Input: part model. Units: mm. Frame: model coordinates. Round coordinates to 2 decimals unless told otherwise and drop trailing zeros. Write each loop counter-clockwise with the first axis right and the second up, starting at its lowest first coordinate (ties: lowest second). Pieces come first, ordered by that corner, then holes. Notation, with made-up numbers: (-1.75, 45.5) - (44.25, 45.5) arc R13 ccw to (44.25, 59.5) - close; hole circle Ø6 at (63, 82.5). An arc over 180 degrees is marked (long way). Use one line per item in the form item = value.
```python
from build123d import *

# Parameters (mm, degrees)
BOSS_EXTRUDE1_DEPTH = 3.175
FILLET1_R           = 50.8
SKETCH2_R           = 3.175
CUT_EXTRUDE1_DEPTH  = 131.731020699
SKETCH3_R           = 2.38125
CUT_EXTRUDE2_DEPTH  = 131.731020699
SKETCH4_W           = 148.329762774
SKETCH4_H           = 42.508472293
CUT_EXTRUDE3_DEPTH  = 131.731020699


with BuildPart() as part:
    # Sketch1 → Boss-Extrude1 (new body)
    with BuildSketch(Plane.XY):
        Polygon((12.7, -76.2), (12.7, 25.4), (-25.408227408, 101.6), (-82.206807187, 101.6), (-12.7, -37.383601913), (-12.7, -76.2), align=None)
    extrude(amount=BOSS_EXTRUDE1_DEPTH)

    # Fillet1
    fillet1_edges = [part.edges().sort_by_distance(p)[0] for p in [
        (-12.7, -37.383601913, 1.5875),
    ]]
    fillet(fillet1_edges, radius=FILLET1_R)

    # Sketch2 → Cut-Extrude1 (cut, through all)
    with BuildSketch(Plane(origin=(0, 0, 0), x_dir=(-1, 0, 0), z_dir=(0, 0, -1))):
        with Locations((0, -63.5)):
            Circle(SKETCH2_R)
        with Locations((0, -38.1)):
            Circle(SKETCH2_R)
        with Locations((0, -12.7)):
            Circle(SKETCH2_R)
        with Locations((0, 12.7)):
            Circle(SKETCH2_R)
    extrude(amount=-CUT_EXTRUDE1_DEPTH, mode=Mode.SUBTRACT)

    # Sketch3 → Cut-Extrude2 (cut, through all)
    with BuildSketch(Plane(origin=(0, 0, 0), x_dir=(-1, 0, 0), z_dir=(0, 0, -1))):
        with Locations((33.256501118, 88.9)):
            Circle(SKETCH3_R)
        with Locations((61.655791008, 88.9)):
            Circle(SKETCH3_R)
        with Locations((19.055016681, 60.503163208)):
            Circle(SKETCH3_R)
        with Locations((47.45430657, 60.503163208)):
            Circle(SKETCH3_R)
        with Locations((4.853532243, 32.106326416)):
            Circle(SKETCH3_R)
        with Locations((33.252822133, 32.106326416)):
            Circle(SKETCH3_R)
    extrude(amount=-CUT_EXTRUDE2_DEPTH, mode=Mode.SUBTRACT)

    # Sketch4 → Cut-Extrude3 (cut, through all)
    with BuildSketch(Plane(origin=(0, 0, 0), x_dir=(-1, 0, 0), z_dir=(0, 0, -1))):
        with Locations((56.905806916, 97.454236147)):
            Rectangle(SKETCH4_W, SKETCH4_H)
    extrude(amount=-CUT_EXTRUDE3_DEPTH, mode=Mode.SUBTRACT)


solid = part.part
```
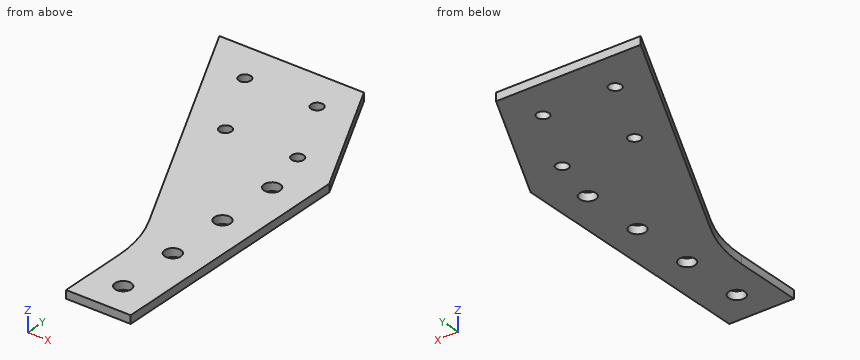
(1) Cut plane C-C on z = 1.2. Count the separate pieces of the cut face and the enclosed holes in it, then the cut area to 3 significant figures.
Derived:
separate_pieces = 1
enclosed_holes = 8
area = 6,260 mm^2
(2) Cut plane A-A on y = -63.5. Output: boundary loops of the cut face in (x, z) (3 decimals), then the cut area to 3 significant figures.
Derived:
outline = (-12.7, 0) - (-3.175, 0) - (-3.175, 3.175) - (-12.7, 3.175) - close; (3.175, 0) - (12.7, 0) - (12.7, 3.175) - (3.175, 3.175) - close
area = 60.5 mm^2
(3) Cut plane D-D on y = 12.7. Output: boundary loops of the cut face in (x, z) (3 decimals).
Derived:
outline = (-37.747, 0) - (-3.175, 0) - (-3.175, 3.175) - (-37.747, 3.175) - close; (3.175, 0) - (12.7, 0) - (12.7, 3.175) - (3.175, 3.175) - close
(4) First-contact query: pin 1 Ø4 at (x, y) = (-47.45, 60.5) entering from +Z; pin 2 Ø1.5 at (y, z) = (56, 2) entering from +X; pin 3 Ø1 at (y, z) = (-68, 1) entering from -X. Flat tips, straight axial feed; report the tip coordinate or a pass-through.
Derived:
pin_1 = through
pin_2 = -2.23
pin_3 = -12.7
(5) Cut plane B-B on x = -1. Output: boundary loops of the cut face in (y, z) (3 decimals).
Derived:
outline = (-76.2, 0) - (-66.513, 0) - (-66.513, 3.175) - (-76.2, 3.175) - close; (-60.487, 0) - (-41.113, 0) - (-41.113, 3.175) - (-60.487, 3.175) - close; (-35.087, 0) - (-15.713, 0) - (-15.713, 3.175) - (-35.087, 3.175) - close; (-9.687, 0) - (9.687, 0) - (9.687, 3.175) - (-9.687, 3.175) - close; (15.713, 0) - (52.794, 0) - (52.794, 3.175) - (15.713, 3.175) - close
(6) Material intervals for L1, parallel to X at y = 59, z = 2.65; L2, parallel to X at y = -57.5, z = 2; L3, parallel to Y at x = 0, z = 2.2 (3 decimals), sorted ascending.
Derived:
L1 = -60.9 to -49.3, -45.61 to -20.9, -17.21 to -4.1
L2 = -12.7 to 12.7
L3 = -76.2 to -66.675, -60.325 to -41.275, -34.925 to -15.875, -9.525 to 9.525, 15.875 to 50.795
